```python
from build123d import *

# Parameters (mm, degrees)
SKETCH1_W                                      = 43.18
SKETCH1_H                                      = 44.45
BOSS_EXTRUDE1_DEPTH                            = 9.525
SKETCH4_R                                      = 4.7625
CUT_EXTRUDE1_DEPTH                             = 51.32550273
MOTORHOLES_D                                   = 2.2606
MOTORHOLES_DEPTH                               = 6.35
MOTORHOLES_TIP                                 = 0.679152758
CBORE_FOR_6_SOCKET_HEAD_CAP_SCREW1_D           = 3.6576
CBORE_FOR_6_SOCKET_HEAD_CAP_SCREW1_CBORE_D     = 7.14502
CBORE_FOR_6_SOCKET_HEAD_CAP_SCREW1_CBORE_DEPTH = 3.5052


with BuildPart() as part:
    # Sketch1 → Boss-Extrude1 (new body)
    with BuildSketch(Plane(origin=(0, 0, 0), x_dir=(1, 0, 0), z_dir=(0, 1, 0))):
        Rectangle(SKETCH1_W, SKETCH1_H)
    extrude(amount=BOSS_EXTRUDE1_DEPTH)

    # Sketch4 → Cut-Extrude1 (cut, through all)
    with BuildSketch(Plane.XY.offset(22.225)):
        with Locations((0, 9.525)):
            Circle(SKETCH4_R)
    extrude(amount=-CUT_EXTRUDE1_DEPTH, mode=Mode.SUBTRACT)

    # MotorHoles
    with Locations(Plane(origin=(0, 0, 0), x_dir=(-1, 0, 0), z_dir=(0, -1, 0))):
        with Locations((-5.715, -19.05), (5.715, -19.05), (13.081, 19.9644), (-13.081, 19.9644)):
            Hole(MOTORHOLES_D / 2, depth=MOTORHOLES_DEPTH)
            with Locations((0, 0, -(MOTORHOLES_DEPTH + MOTORHOLES_TIP / 2))):  # 118° drill point
                Cone(0, MOTORHOLES_D / 2, MOTORHOLES_TIP, mode=Mode.SUBTRACT)

    # CBORE for #6 Socket Head Cap Screw1 (through all)
    with Locations(Plane(origin=(0, 0, 0), x_dir=(-1, 0, 0), z_dir=(0, -1, 0))):
        with Locations((-15.875, 9.525), (15.875, 9.525)):
            CounterBoreHole(CBORE_FOR_6_SOCKET_HEAD_CAP_SCREW1_D / 2, CBORE_FOR_6_SOCKET_HEAD_CAP_SCREW1_CBORE_D / 2, CBORE_FOR_6_SOCKET_HEAD_CAP_SCREW1_CBORE_DEPTH)


solid = part.part
```
Model file for the job. Use its own axes, mm. A direction names the side the tool comes from. Coordinates: 2 decimals unless noted, no trailing zeros. Write each loop counter-clockwise with the first axis right and the second up, starting at its lowest first coordinate (ties: lowest second). Pieces come first, ordered by that corner, then holes. Notation, with made-up numbers: (67, 16.5) - (103, 16.5) arc R27 ccw to (103, 43.5) - close; hole circle Ø9 at (-13.5, -25.75). An arc over 180 degrees is marked (long way). One line per item, written item: value. Start each with the question number.
1. Flat gauge pins, fed straight in: pin 1 (2 mm diameter, centred on x = 13.08, z = -19.96, fed in from -Y); pin 2 (3.5 mm diameter, centred on x = -16, z = -9.5, fed in from -Y). Where does each tip first touch, or does it go through?
2. Slice it at C-C (x = -16). Write the cut outline in (y, z) (3 decimals), plus the area to 3 significant figures.
3. Slice it at A-A (y = 1). Count the separate pieces of the cut face and the enclosed holes in it, plus the area to 3 significant figures.
4. Tool access for faces 1 (the flat face through (-13, 9.525, 0)), 2 (the cylindrical face through (18.51, 1.73, -11.94)): list every direction of +Z, -Z, +X, -X, +Y, -Y with a clear straight run to the whole face (end or side of a thin tool).
5. Slice it at D-D (z = -6.5). Write the cut outline in (x, y) (1 decimal).
6. Probe line 1 (X direction, y = 1, z = -20); line 2 (X direction, y = 3.5, z = -19); line 3 (X direction, y = 9.25, z = -13). List the from-to ranges inside material, lowest first. Write a range as from..to.
7. Slice it at B-B (z = 11). Write the cut outline in (x, y) (1 decimal).
8. Mould opens along X. For faces 3 (the flat face through (13, 9.525, 0)), 4 (the flat face through (21.59, 5, 0)), 5 (the cylindrical face through (-15.031, 6.557, -7.903)), 6 (the flat face through (-21.59, 5, 0)) say: released by +X, released by -X, zero draft, split by the parting line, or undercut.
Answers below:
1. pin 1: stops at y = 6.43
1. pin 2: stops at y = 3.51
2. outline: (0, -22.225) - (9.525, -22.225) - (9.525, -11.35) - (3.505, -11.35) - (3.505, -13.095) - (0, -13.095) - close; (0, -5.955) - (3.505, -5.955) - (3.505, -7.7) - (9.525, -7.7) - (9.525, 22.225) - (0, 22.225) - close
2. area: 376 mm^2
3. separate pieces: 1
3. enclosed holes: 6
3. area: 1,820 mm^2
4. face 1: +Z, -Z, +X, -X, +Y
4. face 2: -Y
5. outline: (-21.6, 0) - (-17.8, 0) - (-17.8, 3.5) - (-14, 3.5) - (-14, 0) - (14, 0) - (14, 3.5) - (17.8, 3.5) - (17.8, 0) - (21.6, 0) - (21.6, 9.5) - (4.8, 9.5) arc R4.8 cw to (-4.8, 9.5) - (-21.6, 9.5) - close
6. line 1: x = -21.59..-14.21, -11.95..11.95, 14.21..21.59
6. line 2: x = -21.59..-13.67, -12.49..12.49, 13.67..21.59
6. line 3: x = -21.59..-4.75, 4.75..21.59
7. outline: (-21.6, 0) - (21.6, 0) - (21.6, 9.5) - (4.8, 9.5) arc R4.8 cw to (-4.8, 9.5) - (-21.6, 9.5) - close
8. face 3: zero draft
8. face 4: released by +X
8. face 5: undercut
8. face 6: released by -X
